Read the model definition and answer for the solid it produces. Units are mm, in the model's axes. Face numbers are marked on the shaded views. A direction names the side the tool comes from. Coordinates: 2 decimals unless noted, no trailing zeros. Loops run counter-clockwise (first coordinate to the right, second up) from the corner with the lowest first, then second, coordinate; pieces in that order, holes last. Notation, with made-up numbers: (11, 64.5) - (40, 64.5) arc R12 ccw to (40, 81.5) - close; hole circle Ø9 at (39, -17.75). An arc over 180 degrees is marked (long way). Use one line per item in the form item = value.
from build123d import *

# Parameters (mm, degrees)
SKETCH_1_R          = 3
EXTRUDE_1_DEPTH     = 2.8
SKETCH_2_R          = 1.4
CUT_EXTRUDE_1_DEPTH = 6.083306011
SKETCH_3_OUTSIDE_W  = 9.788
SKETCH_3_OUTSIDE_H  = 9.788
SKETCH_3_OUTSIDE_R  = 1.7
CUT_EXTRUDE_2_DEPTH = 1.8


with BuildPart() as part:
    # 草图1 → 拉伸1 (new body)
    with BuildSketch(Plane(origin=(0, 0, 0), x_dir=(1, 0, 0), z_dir=(0, 1, 0))):
        with Locations(Location((0, 0, 0), (0, 0, 270))):
            Circle(SKETCH_1_R)
    extrude(amount=EXTRUDE_1_DEPTH)

    # 草图2 → 切除-拉伸1 (cut, through all)
    with BuildSketch(Plane(origin=(0, 2.8, 0), x_dir=(-1, 0, 0), z_dir=(0, 1, 0))):
        with Locations(Location((0, 0, 0), (0, 0, 90))):
            Circle(SKETCH_2_R)
    extrude(amount=-CUT_EXTRUDE_1_DEPTH, mode=Mode.SUBTRACT)

    # 草图3 outside → 切除-拉伸2 (cut)
    with BuildSketch(Plane(origin=(0, 2.8, 0), x_dir=(1, 0, 0), z_dir=(0, 1, 0))):
        Rectangle(SKETCH_3_OUTSIDE_W, SKETCH_3_OUTSIDE_H)
        with Locations(Location((0, 0, 0), (0, 0, 270))):
            Circle(SKETCH_3_OUTSIDE_R, mode=Mode.SUBTRACT)
    extrude(amount=-CUT_EXTRUDE_2_DEPTH, mode=Mode.SUBTRACT)


solid = part.part
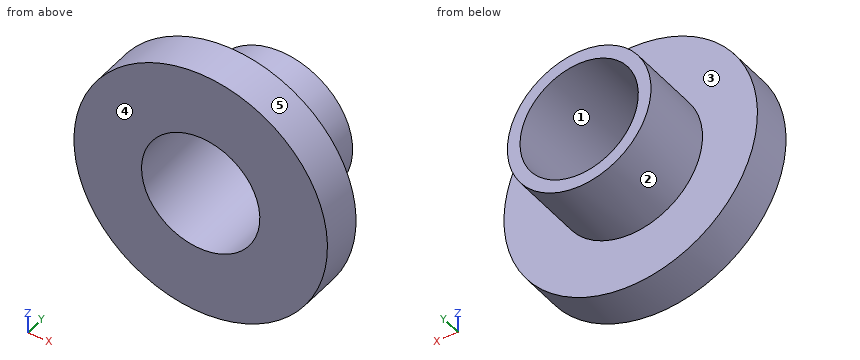
Item 1: The part is cut by section A-A on x = 0. Give the vertices of the cut face in (y, z), plus the area to 3 significant figures.
Results below:
outline = (0, -3) - (1, -3) - (1, -1.7) - (2.8, -1.7) - (2.8, -1.4) - (0, -1.4) - close; (0, 1.4) - (2.8, 1.4) - (2.8, 1.7) - (1, 1.7) - (1, 3) - (0, 3) - close
area = 4.28 mm²
Item 2: The part is cut by section C-C on y = 2.15. Give the vertices of the cut face in (x, z), plus the area to 3 significant figures.
Results below:
outline = circle Ø3.4 at (0, 0); hole circle Ø2.8 at (0, 0)
area = 2.92 mm²
Item 3: This flat-tipped pin is pushed along its axis until it touches: P1, Ø1.5, axis at x = -2.5, z = -0.5, coming from the +Y side. Where does it stop, or does it pass through?
Results below:
P1 = 1
Item 4: The part is cut by section D-D on x = 1.55. Give the vertices of the cut face in (y, z).
Results below:
outline = (0, -2.57) - (1, -2.57) - (1, -0.7) - (2.8, -0.7) - (2.8, 0.7) - (1, 0.7) - (1, 2.57) - (0, 2.57) - close
Item 5: Find the intervals of material crossed by L1, parallel to X at y = 1.95, z = 0; L2, parallel to X at y = 0.85, z = 0; L3, parallel to Y at x = 2.05, z = 0, in increasing order.
Results below:
L1 = -1.7 to -1.4, 1.4 to 1.7
L2 = -3 to -1.4, 1.4 to 3
L3 = 0 to 1
Item 6: The part is cut by section B-B on z = 0. Give the vertices of the cut face in (x, y).
Results below:
outline = (-3, 0) - (-1.4, 0) - (-1.4, 2.8) - (-1.7, 2.8) - (-1.7, 1) - (-3, 1) - close; (1.4, 0) - (3, 0) - (3, 1) - (1.7, 1) - (1.7, 2.8) - (1.4, 2.8) - close
Item 7: For a pull along Y with two mould halves and no side action, classify the marked faces 3, 4 and 5 as +Y half, -Y half, draft (parallel to the pull), parting line (faces both ways), or undercut.
Results below:
face_3 = +Y half
face_4 = -Y half
face_5 = draft
Item 8: Which of the six approach directions +Z, -Z, +X, -X, +Y, -Y give full straight-line access (tool end or side, diameter ignored) to the marked faces 1 and 2?
Results below:
face_1 = +Y, -Y
face_2 = +Y
